```python
from build123d import *


with BuildPart() as part:
    # Croquis1 → Revolución1 (revolve)
    with BuildSketch(Plane.XY, mode=Mode.PRIVATE) as revoluci_n1_sk:
        with BuildLine():
            Line((10.846100741, 34.389443091), (14.068704784, 35.913637022))
            ThreePointArc((14.068704784, 35.913637022), (14.638684043, 36.747496005), (14.19097791, 37.652899991))
            Line((14.19097791, 37.652899991), (11.384961428, 39.5))
            Line((11.384961428, 39.5), (11.384961428, 40))
            Line((11.384961428, 40), (37.307240053, 40))
            Line((37.307240053, 40), (37.307240053, 39.5))
            Line((37.307240053, 39.5), (34.501223571, 37.652899991))
            ThreePointArc((34.501223571, 37.652899991), (34.053517438, 36.747496005), (34.623496697, 35.913637022))
            Line((34.623496697, 35.913637022), (37.846100741, 34.389443091))
            Line((37.846100741, 34.389443091), (37.846100741, 33))
            Line((37.846100741, 33), (31.846100741, 33))
            Line((31.846100741, 33), (31.846100741, 39.5))
            Line((31.846100741, 39.5), (29.346100741, 39.5))
            Line((29.346100741, 39.5), (29.346100741, 37))
            Line((29.346100741, 37), (19.346100741, 37))
            Line((19.346100741, 37), (19.346100741, 39.5))
            Line((19.346100741, 39.5), (16.846100741, 39.5))
            Line((16.846100741, 39.5), (16.846100741, 33))
            Line((16.846100741, 33), (10.846100741, 33))
            Line((10.846100741, 33), (10.846100741, 34.389443091))
        make_face()
    revolve(revoluci_n1_sk.sketch.rotate(Axis((0, 0, 0), (1, 0, 0)), 90), axis=Axis((0, 0, 0), (1, 0, 0)))


solid = part.part
```
Geometry check sheet. Reference: the model listing, model coordinates, mm. A direction names the side the tool comes from. Coordinates: 2 decimals unless noted, no trailing zeros. Order: outer loops, then holes, each group sorted by start corner. A loop starts at its lowest first (then second) coordinate and runs counter-clockwise, first axis right, second up. Notation, with made-up numbers: (-1, 3) - (28, 3) arc R11 ccw to (28, 8) - close; hole circle Ø6 at (72.5, 47.5). An arc over 180 degrees is marked (long way). Use one line per item in the form item = value.
1. Section check A-A (x = 24.75). Record the boundary of the cut face in (y, z).
Here are the results:
outline = circle Ø80 at (0, 0); hole circle Ø74 at (0, 0)
2. Access from +Z, -Z, +X, -X, +Y, -Y to the whole of each face (thin tool, end or side, straight path). Record for faces 5 (the face through (11.385, 35.4, 18)), 6 (the face through (30.579, -11.865, 37.676)), 7 (the face through (37.307, -18, 35.4)).
Here are the results:
face_5 = -X
face_6 = none
face_7 = +X
3. Draft check along X on faces 1 (the face through (13.804, -9.912, 31.476)), 2 (the face through (31.846, 32, 9)), 3 (the face through (10.846, -13, 31)), 4 (the face through (18.079, -11.865, 37.676)). Enter one of: pulls with the +X half, pulls with the -X half, needs draft (parallel to the pull), parting line crosses it, or undercut.
Here are the results:
face_1 = needs draft
face_2 = undercut
face_3 = pulls with the -X half
face_4 = undercut
4. Gauge pin test, flat ends, axial feed: pin 1 (6 mm diameter, centred on x = 27.5, z = -5, fed in from -Y); pin 2 (10 mm diameter, centred on y = 21.5, z = -10, fed in from -X); pin 3 (6 mm diameter, centred on x = 18, y = -15, fed in from -Z); pin 4 (2 mm diameter, centred on x = 26, z = -6, fed in from -Y). Record the tip position at first contact, or that the pin passes through.
Here are the results:
pin_1 = -39.95
pin_2 = through
pin_3 = -38.16
pin_4 = -39.69
5. Scan lines: line 1 (X direction, y = -5, z = 37.5); line 2 (Y direction, x = 13.75, z = -18); line 3 (X direction, y = -17.5, z = -28.5). Record each from-to range of solid material in increasing order.
Here are the results:
line_1 = 13.92 to 16.85, 19.35 to 29.35, 31.85 to 34.77
line_2 = -35.72 to -33.4, -30.9 to -27.66, 27.66 to 30.9, 33.4 to 35.72
line_3 = 10.85 to 16.85, 31.85 to 37.85
